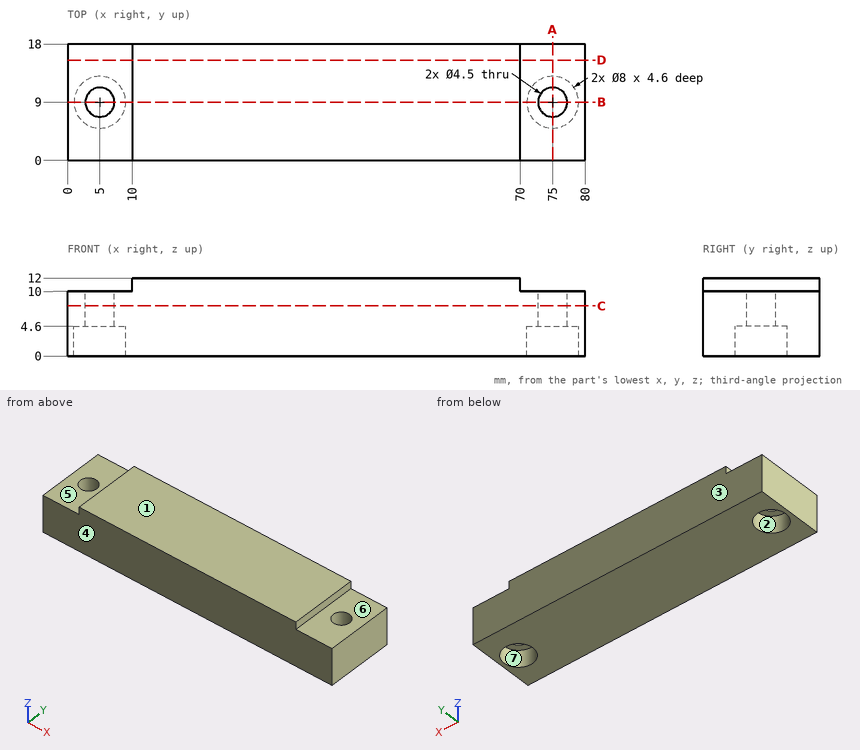
Check sheet for the drawn part. Datum: minimum x, y, z corner. Units: mm. A direction names the side the tool comes from. Give positions to 0.01 mm unless a question says otherwise; leave off trailing zeros. Write each loop counter-clockwise with the first axis right and the second up, starting at its lowest first coordinate (ties: lowest second). Pieces come first, ordered by that corner, then holes. Notation, with made-up numbers: M 35.25,46 L 49.25,46 A12 ccw 49.25,60 Z; hole C 85,70 d1. An arc over 180 degrees is marked long. Write item = value, one per line.
(1) Draft check along Y on the marked faces 1, 2, 3 and 4. Enter one of: released by +Y, released by -Y, zero draft, split by the parting line, or undercut.
Found:
face_1 = zero draft
face_2 = undercut
face_3 = released by +Y
face_4 = released by -Y
(2) Sectioned sample at B-B (y = 9). Record the cut outline in (x, z), then the cut area to 3 significant figures.
Found:
outline = M 0,0 L 1,0 L 1,4.6 L 2.75,4.6 L 2.75,10 L 0,10 Z; M 7.25,4.6 L 9,4.6 L 9,0 L 71,0 L 71,4.6 L 72.75,4.6 L 72.75,10 L 70,10 L 70,12 L 10,12 L 10,10 L 7.25,10 Z; M 77.25,4.6 L 79,4.6 L 79,0 L 80,0 L 80,10 L 77.25,10 Z
area = 798 mm2
(3) Go/stop test with flat-tipped pins: pin 1 Ø7 at (x, y) = (5, 9) entering from +Z; pin 2 Ø4 at (x, y) = (74, 10) entering from -Z; pin 3 Ø1.6 at (y, z) = (12, 11) entering from -X. Record where each tip stops, or that it passes through.
Found:
pin_1 = 10
pin_2 = 4.6
pin_3 = 10
(4) Sectioned sample at C-C (z = 7.75). Record the cut outline in (x, y).
Found:
outline = M 0,0 L 80,0 L 80,18 L 0,18 Z; hole C 5,9 d4.5; hole C 75,9 d4.5
(5) Material ranges on line 1 (X direction, y = 9, z = 1.4); line 2 (X direction, y = 9, z = 7.1); line 3 (Y direction, x = 75, z = 1.7), recorded low to high.
Found:
line_1 = 0 to 1, 9 to 71, 79 to 80
line_2 = 0 to 2.75, 7.25 to 72.75, 77.25 to 80
line_3 = 0 to 5, 13 to 18
(6) Access from +Z, -Z, +X, -X, +Y, -Y to the whole of each face (thin tool, end or side, straight path). Record for the marked faces 5, 6 and 7.
Found:
face_5 = +Z, -X, +Y, -Y
face_6 = +Z, +X, +Y, -Y
face_7 = -Z
(7) Sectioned sample at A-A (x = 75). Record the cut outline in (y, z).
Found:
outline = M 0,0 L 5,0 L 5,4.6 L 6.75,4.6 L 6.75,10 L 0,10 Z; M 11.25,4.6 L 13,4.6 L 13,0 L 18,0 L 18,10 L 11.25,10 Z
(8) Sectioned sample at D-D (y = 15.5). Record the cut outline in (x, z).
Found:
outline = M 0,0 L 80,0 L 80,10 L 70,10 L 70,12 L 10,12 L 10,10 L 0,10 Z
